Here's how the part is built. I have some questions about the finished solid (model axes, mm). A direction names the side the tool comes from. Round coordinates to 2 decimals unless told otherwise and drop trailing zeros. Loops run counter-clockwise (first coordinate to the right, second up) from the corner with the lowest first, then second, coordinate; pieces in that order, holes last. Notation, with made-up numbers: (-22, 14) -> (-18, 14) arc R17 ccw to (-18, 36) -> close; hole circle Ø2 at (37.5, 39.25). An arc over 180 degrees is marked (long way). Use CSV: the item, a comma, the result in double quotes. Start each with the question number.
Autodesk Inventor part; units mm, degrees
ref_plane "YZ Plane" through (0, 0, 0) normal (1, 0, 0) x (0, 1, 0)
ref_plane "XZ Plane" through (0, 0, 0) normal (0, 1, 0) x (-1, 0, 0)
ref_plane "XY Plane" through (0, 0, 0) normal (0, 0, 1) x (1, 0, 0)
sketch "Sketch1" plane through (0, 0, 0) normal (0, 1, 0) x (-1, 0, 0)
  circle A0 centre (0, 0) radius 10
  circle A1 centre (-54, 0) radius 10
  line L0 (-54, -10) -> (0, -10)
  line L1 (0, 10) -> (-54, 10)
  circle A2 centre (-16, -6.1173) radius 1.25
  circle A3 centre (-37, -6.1173) radius 1.25
  circle A4 centre (-37, 6.3827) radius 1.25
  circle A5 centre (-16, 6.3827) radius 1.25
  line L2 (-11, -10) -> (-11, 10)
  line L3 (-21, 10) -> (-21, -10)
  line L4 (-32, -10) -> (-32, 10)
  line L5 (-42, -10) -> (-42, 10)
  line L6 (13, -20) -> (-67, -20)
  line L7 (-67, -20) -> (-67, 20)
  line L8 (-67, 20) -> (13, 20)
  line L9 (13, 20) -> (13, -20)
  dimension "d0" = 20
  dimension "d1" = 20
  dimension "d2" = 54
  dimension "d3" = 21
  dimension "d4" = 12.5
  dimension "d5" = 12.5
  dimension "d6" = 21
  dimension "d7" = 2.5
  dimension "d8" = 2.5
  dimension "d9" = 2.5
  dimension "d10" = 2.5
  dimension "d11" = 5
  dimension "d12" = 5
  dimension "d13" = 5
  dimension "d14" = 5
  dimension "d15" = 11
  dimension "d16" = 11
  dimension "d17" = 40
  dimension "d18" = 80
  dimension "d19" = 13
  dimension "d20" = 20
extrude "Extrusion1" add sketch "Sketch1" along normal blind 5 contours L2 L0 L3 L1 | L4 L0 L5 L1 | L6 L7 L8 L9
sketch "Sketch2" plane through (67, 0, 20) normal (1, 0, 0) x (0, 0, -1)
  line L0 (0, 0) -> (-17.6204, 0)
  line L1 (-17.6204, 0) -> (-17.6204, 5)
  line L2 (-17.6204, 5) -> (0, 5)
  line L3 (0, 5) -> (0, 0)
  line L4 (-17.6204, 5) -> (13.1355, 35.7559)
  line L5 (13.1355, 35.7559) -> (9.5999, 39.2914)
  line L6 (9.5999, 39.2914) -> (-22.6204, 7.0711)
  line L7 (-22.6204, 7.0711) -> (-22.6204, 0)
  line L8 (-22.6204, 0) -> (-17.6204, 0)
  circle A0 centre (-22.6204, 3.5355) radius 3.5355
  point P0 (-22.6204, 0)
  dimension "d23" = 45
  dimension "d24" = 5
  dimension "d25" = 5
extrude "Extrusion2" add sketch "Sketch2" against normal blind 80
sketch "Sketch3" plane through (0, 5, 0) normal (0, 1, 0) x (1, 0, 0)
  line L0 (12, -20) -> (42, -20)
  line L1 (42, -20) -> (42, -30)
  line L2 (42, -30) -> (12, -30)
  line L3 (12, -30) -> (12, -20)
  line L4 (-13, 20) -> (-13, -37.6204)
  line L5 (11, -10) -> (0, -10)
  point P0 (0, 0)
  dimension "d28" = 30
  dimension "d29" = 10
  dimension "d30" = 25
  dimension "d31" = 10
extrude "Extrusion3" cut sketch "Sketch3" against normal blind 80
sketch "Sketch4" plane through (67, 5, 37.6204) normal (0, -0.7071, -0.7071) x (-1, 0, 0)
  circle A0 centre (73.7126, 34.5024) radius 2.2513
  circle A1 centre (10, 33.4954) radius 2.25
  line L0 (0, 0) -> (0, 43.4954)
  line L1 (0, 43.4954) -> (80, 43.4954)
  circle A2 centre (70, 33.4954) radius 2.25
  line L2 (80, 37.2082) -> (80, -7.0711)
  point P0 (67, 23.0661)
  point P1 (71.5496, 35.1267)
  point P2 (72.1615, 32.8706)
  dimension "d34" = 10
  dimension "d35" = 10
  dimension "d36" = 4.5
  dimension "d37" = 10
  dimension "d38" = 10
  dimension "d39" = 4.5
extrude "Extrusion4" cut sketch "Sketch4" against normal blind 80 contours A2 A0 | A0 A2 | A1 picked at (71.7698, 33.9272) picked at (69.1023, 33.1672)
sketch "Sketch5" plane through (0, 0, 0) normal (0, -1, 0) x (1, 0, 0)
  line L0 (42, 10) -> (42, -10)
  circle A0 centre (42, -10) radius 3.5
  circle A1 centre (42, 10) radius 3.5
  line L1 (11, -10) -> (11, 10)
  circle A2 centre (11, 10) radius 3.5
  circle A3 centre (11, -10) radius 3.5
  line L2 (0, -10) -> (11, -10)
  line L3 (42, -10) -> (54, -10)
  circle A4 centre (42, -6.5) radius 3.5
  circle A5 centre (42, 6.5) radius 3.5
  circle A6 centre (11, 6.5) radius 3.5
  circle A7 centre (11, -6.5) radius 3.5
  line L4 (14.5, -6.5) -> (14.5, -6.5)
  line L5 (14.5, -6.5) -> (14.5, -10)
  line L6 (14.5, -10) -> (14.5, -10)
  line L7 (14.5, -10) -> (14.5, -6.5)
  line L8 (14.5, 10) -> (14.5, 6.5)
  line L9 (38.5, -10) -> (38.5, -6.5)
  line L10 (38.5, 10) -> (38.5, 6.5)
  point P0 (0, 0)
  point P1 (11, -3)
  point P2 (11, 6.5)
  point P3 (42, 9)
  point P4 (42, -3)
  point P5 (7.5, -10)
  point P6 (45.5, -10)
  point P7 (7.9689, 8.25)
  point P8 (7.9689, -8.25)
  point P9 (42, -3)
  point P10 (45.0311, 8.25)
  dimension "d42" = 7
  dimension "d43" = 7
  dimension "d44" = 7
  dimension "d45" = 7
  dimension "d46" = 20
  dimension "d47" = 0
  dimension "d48" = 20
  dimension "d49" = 0
extrude "Extrusion5" cut sketch "Sketch5" against normal blind 6 contours A5 A1 L0 | A5 A1 | L0 A1 A5 | A1 A5 L0 | L0 A5 A1 | L0 A0 A4 | A5 L10 A1 | A0 A4 L0 | L0 A4 A0 | A4 A0 L9 | A4 A0 L3 | L3 A0 A4 | A7 A3 L1 | A7 A3 L2 | L2 A3 A7 | L1 A3 A7 | A3 A7 L1 | L1 A7 A3 | A6 A2 L1 | L1 A2 A6 | A7 L5 A3 | A2 A6 L1 | L1 A6 A2 | A2 A6 | A6 A2 L8 picked at (41.7404, -4.1959) picked at (42.2426, -8.8078) picked at (41.7574, -7.6922)
equation "\"d5\" = d4"
equation "\"d6\" = d3"
equation "\"d39\" = d36"
equation "\"d43\" = d42"
equation "\"d44\" = d42"
equation "\"d45\" = d42"
properties part number "CameraBracket"
Q1. Will these pins go through, and if not, where does the flat tip stop? pin 1 Ø5 at (x, y) = (11.5, 31.5) entering from -Z; pin 2 Ø20 at (x, z) = (10, -3.5) entering from +Y; pin 3 Ø4 at (x, y) = (35, 31.5) entering from -Z.
Q2. If we mould it in two halves opening along Z, with no side actions, what happens to faces 1 (the flat face through (27.56, 20.16, 22.46)), 2 (the flat face through (27, 3, 30))? For each: pulls with the +Z half, pulls with the -Z half, needs draft (parallel to the pull), parting line crosses it, or undercut.
Q3. I want a section at C-C, the plane z = 31.5. List the corners of the cut face in (x, y) for me, then the cut area to 3 significant figures.
Q4. I want a section at B-B, the plane x = 49.5. List the corners of the cut face in (y, z) for me.
Q5. I need wall thicknesses on line 1 along Z through (x, y) = (37, 3); line 2 along Z through (x, y) = (16, 1.35); line 3 along Y through (x, z) = (20.5, -16). Which ranges of each line are inside material? Lowest first, please.
Q6. I want a section at D-D, the plane x = 16. List the corners of the cut face in (y, z) for me.
Q7. I want a section at A-A, the plane z = 0. List the corners of the cut face in (x, y) for me, then the cut area to 3 significant figures.
Q8. For faces 3 (the flat face through (27, 3, 20)), 4 (the flat face through (26, 2, -20)), 5 (the cylindrical face through (13.45, 2.46, 4)), which set-ups out of +Z, -Z, +X, -X, +Y, -Y let a thin tool reach every point of the face, with its end or its side?
Values found:
1,pin 1,"z = 8.62"
1,pin 2,"y = 5"
1,pin 3,"z = 9.12"
2,face 1,"pulls with the -Z half"
2,face 2,"undercut"
3,outline,"(-13, 0) -> (67, 0) -> (67, 5) -> (-13, 5) -> close; (-13, 11.12) -> (67, 11.12) -> (67, 18.19) -> (-13, 18.19) -> close"
3,area,"966 mm2"
4,outline,"(0, -20) -> (5, -20) -> (5, -10) -> (0, -10) -> close; (0, 10) -> (5, 10) -> (5, 37.62) -> (35.76, 6.86) -> (39.29, 10.4) -> (7.07, 42.62) arc R3.54 ccw to (0, 42.62) -> close"
5,line 1,"-20 to -7.37, -4.87 to 5.13, 7.63 to 20, 30 to 46.12"
5,line 2,"-20 to -7.37, -4.87 to 5.13, 7.63 to 20, 30 to 45.4"
5,line 3,"0 to 5"
6,outline,"(0, -20) -> (5, -20) -> (5, -7.37) -> (0, -7.37) -> close; (0, -4.87) -> (5, -4.87) -> (5, 5.13) -> (0, 5.13) -> close; (0, 7.63) -> (5, 7.63) -> (5, 20) -> (0, 20) -> close; (0, 30) -> (5, 30) -> (5, 37.62) -> (35.76, 6.86) -> (39.29, 10.4) -> (7.07, 42.62) arc R3.54 ccw to (0, 42.62) -> close"
7,outline,"(-13, 0) -> (-10, 0) -> (-10, 5) -> (-13, 5) -> close; (11, 0) -> (21, 0) -> (21, 5) -> (11, 5) -> close; (32, 0) -> (42, 0) -> (42, 5) -> (32, 5) -> close; (64, 0) -> (67, 0) -> (67, 5) -> (64, 5) -> close"
7,area,"130 mm2"
8,face 3,"-Y"
8,face 4,"-Z, +X, -X, +Y, -Y"
8,face 5,"+Y, -Y"
